Here's how the part is built. I have some questions about the finished solid (model axes, mm). Give positions to 0.01 mm unless a question says otherwise; leave off trailing zeros. Order: outer loops, then holes, each group sorted by start corner. A loop starts at its lowest first (then second) coordinate and runs counter-clockwise, first axis right, second up.
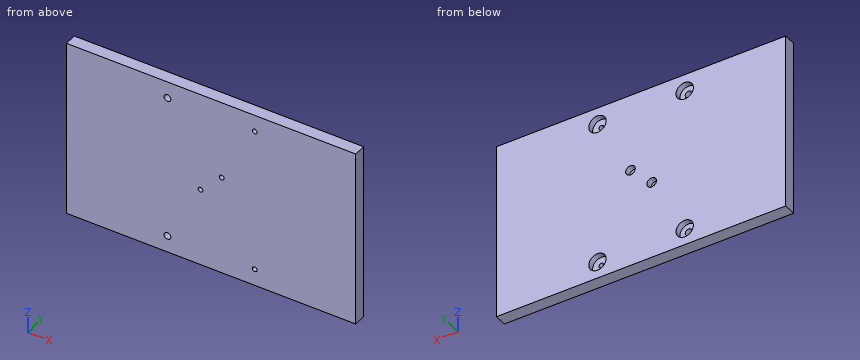
from build123d import *

# Parameters (mm, degrees)
SKETCH1_W           = 300
SKETCH1_H           = 185
SKETCH1_R           = 3.56
SKETCH1_R_2         = 2.5
BOSS_EXTRUDE1_DEPTH = 12.7
CUT_EXTRUDE1_START  = -6.35
SKETCH2_R           = 9
SKETCH2_R_2         = 3.56
SKETCH2_R_3         = 2.5
SKETCH2_R_4         = 5
CUT_EXTRUDE1_DEPTH  = 6.35


with BuildPart() as part:
    # Sketch1 → Boss-Extrude1 (new body)
    with BuildSketch(Plane(origin=(0, 0, 0), x_dir=(1, 0, 0), z_dir=(0, 1, 0))):
        Rectangle(SKETCH1_W, SKETCH1_H)
        with Locations(Location((-45.25, 75, 0), (0, 0, 270))):
            Circle(SKETCH1_R, mode=Mode.SUBTRACT)
        with Locations(Location((-45.25, -75, 0), (0, 0, 270))):
            Circle(SKETCH1_R, mode=Mode.SUBTRACT)
        with Locations(Location((45.25, 75, 0), (0, 0, 270))):
            Circle(SKETCH1_R_2, mode=Mode.SUBTRACT)
        with Locations(Location((45.25, -75, 0), (0, 0, 270))):
            Circle(SKETCH1_R_2, mode=Mode.SUBTRACT)
        with Locations(Location((-11, 11, 0), (0, 0, 270))):
            Circle(SKETCH1_R_2, mode=Mode.SUBTRACT)
        with Locations(Location((11, -11, 0), (0, 0, 270))):
            Circle(SKETCH1_R_2, mode=Mode.SUBTRACT)
    extrude(amount=BOSS_EXTRUDE1_DEPTH)

    # Sketch2 → Cut-Extrude1 (cut)
    # profile 1 of 6: a face of its own
    with BuildSketch(Plane(origin=(0, 12.7, 0), x_dir=(1, 0, 0), z_dir=(0, 1, 0)).offset(CUT_EXTRUDE1_START)):
        with Locations(Location((-45.25, 75, 0), (0, 0, 270))):
            Circle(SKETCH2_R)
        with Locations(Location((-45.25, 75, 0), (0, 0, 270))):
            Circle(SKETCH2_R_2, mode=Mode.SUBTRACT)
    # profile 2 of 6: a face of its own
    with BuildSketch(Plane(origin=(0, 12.7, 0), x_dir=(1, 0, 0), z_dir=(0, 1, 0)).offset(CUT_EXTRUDE1_START)):
        with Locations(Location((45.25, 75, 0), (0, 0, 270))):
            Circle(SKETCH2_R)
        with Locations(Location((45.25, 75, 0), (0, 0, 270))):
            Circle(SKETCH2_R_3, mode=Mode.SUBTRACT)
    # profile 3 of 6: a face of its own
    with BuildSketch(Plane(origin=(0, 12.7, 0), x_dir=(1, 0, 0), z_dir=(0, 1, 0)).offset(CUT_EXTRUDE1_START)):
        with Locations(Location((45.25, -75, 0), (0, 0, 90))):
            Circle(SKETCH2_R)
        with Locations(Location((45.25, -75, 0), (0, 0, 90))):
            Circle(SKETCH2_R_3, mode=Mode.SUBTRACT)
    # profile 4 of 6: a face of its own
    with BuildSketch(Plane(origin=(0, 12.7, 0), x_dir=(1, 0, 0), z_dir=(0, 1, 0)).offset(CUT_EXTRUDE1_START)):
        with Locations(Location((-45.25, -75, 0), (0, 0, 270))):
            Circle(SKETCH2_R)
        with Locations(Location((-45.25, -75, 0), (0, 0, 270))):
            Circle(SKETCH2_R_2, mode=Mode.SUBTRACT)
    # profile 5 of 6: a face of its own
    with BuildSketch(Plane(origin=(0, 12.7, 0), x_dir=(1, 0, 0), z_dir=(0, 1, 0)).offset(CUT_EXTRUDE1_START)):
        with Locations(Location((-11, 11, 0), (0, 0, 270))):
            Circle(SKETCH2_R_4)
        with Locations(Location((-11, 11, 0), (0, 0, 270))):
            Circle(SKETCH2_R_3, mode=Mode.SUBTRACT)
    # profile 6 of 6: a face of its own
    with BuildSketch(Plane(origin=(0, 12.7, 0), x_dir=(1, 0, 0), z_dir=(0, 1, 0)).offset(CUT_EXTRUDE1_START)):
        with Locations(Location((11, -11, 0), (0, 0, 270))):
            Circle(SKETCH2_R_4)
        with Locations(Location((11, -11, 0), (0, 0, 270))):
            Circle(SKETCH2_R_3, mode=Mode.SUBTRACT)
    extrude(amount=CUT_EXTRUDE1_DEPTH, mode=Mode.SUBTRACT)


solid = part.part
Q1. If we section it at A-A on x = -45.25: List the corners of the cut face in (y, z) for me.
Filled sheet:
outline: (0, -92.5) - (12.7, -92.5) - (12.7, -84) - (6.35, -84) - (6.35, -78.56) - (0, -78.56) - close; (0, -71.44) - (6.35, -71.44) - (6.35, -66) - (12.7, -66) - (12.7, 66) - (6.35, 66) - (6.35, 71.44) - (0, 71.44) - close; (0, 78.56) - (6.35, 78.56) - (6.35, 84) - (12.7, 84) - (12.7, 92.5) - (0, 92.5) - close
Q2. I'm going to push flat-ended pins straight in: P1, Ø23.5, axis at x = -45.25, z = -75, coming from the -Y side; P2, Ø8, axis at x = 11, z = 11, coming from the +Y side; P3, Ø3, axis at x = 45.25, z = 75, coming from the +Y side (1 decimal). Where does each tip first touch, or does it pass through?
Filled sheet:
P1: stops at y = 0
P2: stops at y = 6.35
P3: passes through
Q3. If we section it at B-B on y = 9.5: List the corners of the cut face in (x, z) for me.
Filled sheet:
outline: (-150, -92.5) - (150, -92.5) - (150, 92.5) - (-150, 92.5) - close; hole circle Ø18 at (-45.25, -75); hole circle Ø18 at (-45.25, 75); hole circle Ø10 at (-11, -11); hole circle Ø10 at (11, 11); hole circle Ø18 at (45.25, -75); hole circle Ø18 at (45.25, 75)
Q4. I need wall thicknesses on L1, parallel to X at y = 4.25, z = -75; L2, parallel to X at y = 8, z = -75; L3, parallel to Z at x = -49, y = 7.5. Which ranges of each line are inside material? Lowest first, please.
Filled sheet:
L1: x = -150 to -48.81, -41.69 to 42.75, 47.75 to 150
L2: x = -150 to -54.25, -36.25 to 36.25, 54.25 to 150
L3: z = -92.5 to -83.18, -66.82 to 66.82, 83.18 to 92.5
